Input: dimensioned drawing with shaded views. Units: mm. Origin: part minimum x, y, z. A direction names the side the tool comes from. Give positions to 0.01 mm unless a question says otherwise; leave off trailing zeros. Order: outer loops, then holes, each group sorted by start corner. A loop starts at its lowest first (then second) coordinate and runs counter-clockwise, first axis right, second up. Notation, with made-up numbers: (80, -1.75) -> (137, -1.75) arc R7 cw to (137, 7.25) -> close; hole circle Ø4 at (-10, 47). An arc over 180 degrees is marked (long way). Use CSV: the item, a comma, the result in double quotes.
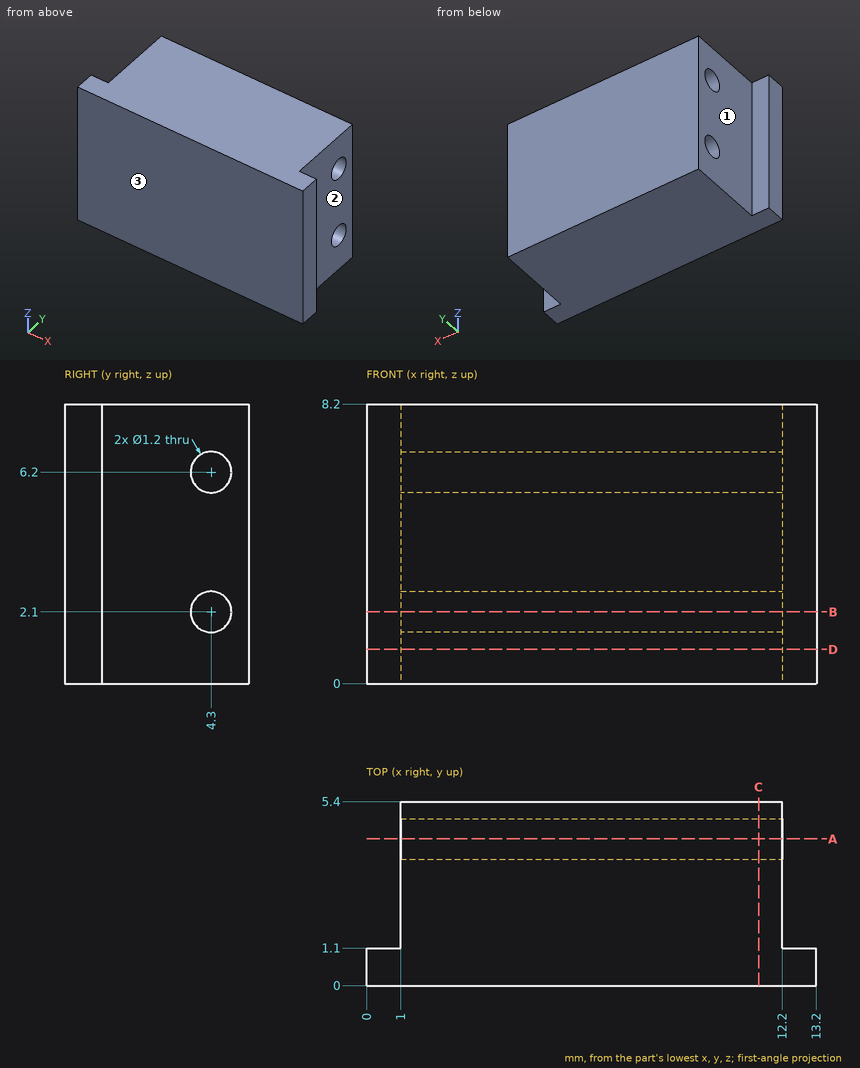
1. Section query B-B on z = 2.1. Return loops of the section in (x, y).
Answer below:
outline,"(0, 0) -> (13.2, 0) -> (13.2, 1.1) -> (12.2, 1.1) -> (12.2, 3.7) -> (1, 3.7) -> (1, 1.1) -> (0, 1.1) -> close; (1, 4.9) -> (12.2, 4.9) -> (12.2, 5.4) -> (1, 5.4) -> close"
2. Access query for the marked faces 1, 2 and 3. Directions: +Z, -Z, +X, -X, +Y, -Y. A direction counts if a zero-diameter tool reaches every point of the face in a straight line with its end or side. Return the directions, or none.
Answer below:
face 1,"+Z, -Z, -X, +Y"
face 2,"+Z, -Z, +X, +Y"
face 3,"+Z, -Z, +X, -X, -Y"
3. Pin query (flat end, axial travel): P1, Ø2, axis at y = 2.5, z = 2.5, coming from the -X side; P2, Ø1.1, axis at y = 4.3, z = 6.2, coming from the -X side; P3, Ø1.6, axis at y = 4.3, z = 2.1, coming from the +X side. Return the tip coordinate at first contact, or that it passes through.
Answer below:
P1,"stops at x = 1"
P2,"passes through"
P3,"stops at x = 12.2"
4. Ray query, line 1 along Y through (x, z) = (7.5, 6.2); line 2 along X through (y, z) = (1.3, 6.5); line 3 along Y through (x, z) = (12.25, 7.25). Return the intervals inside material, ascending.
Answer below:
line 1,"y = 0 to 3.7, 4.9 to 5.4"
line 2,"x = 1 to 12.2"
line 3,"y = 0 to 1.1"
5. Section query A-A on y = 4.3. Return loops of the section in (x, z), plus the area to 3 significant figures.
Answer below:
outline,"(1, 0) -> (12.2, 0) -> (12.2, 1.5) -> (1, 1.5) -> close; (1, 2.7) -> (12.2, 2.7) -> (12.2, 5.6) -> (1, 5.6) -> close; (1, 6.8) -> (12.2, 6.8) -> (12.2, 8.2) -> (1, 8.2) -> close"
area,"65.0 mm²"
6. Section query C-C on x = 11.5. Return loops of the section in (y, z), plus the area to 3 significant figures.
Answer below:
outline,"(0, 0) -> (5.4, 0) -> (5.4, 8.2) -> (0, 8.2) -> close; hole circle Ø1.2 at (4.3, 2.1); hole circle Ø1.2 at (4.3, 6.2)"
area,"42.0 mm²"
7. Section query D-D on z = 1. Return loops of the section in (x, y), plus the area to 3 significant figures.
Answer below:
outline,"(0, 0) -> (13.2, 0) -> (13.2, 1.1) -> (12.2, 1.1) -> (12.2, 5.4) -> (1, 5.4) -> (1, 1.1) -> (0, 1.1) -> close"
area,"62.7 mm²"
